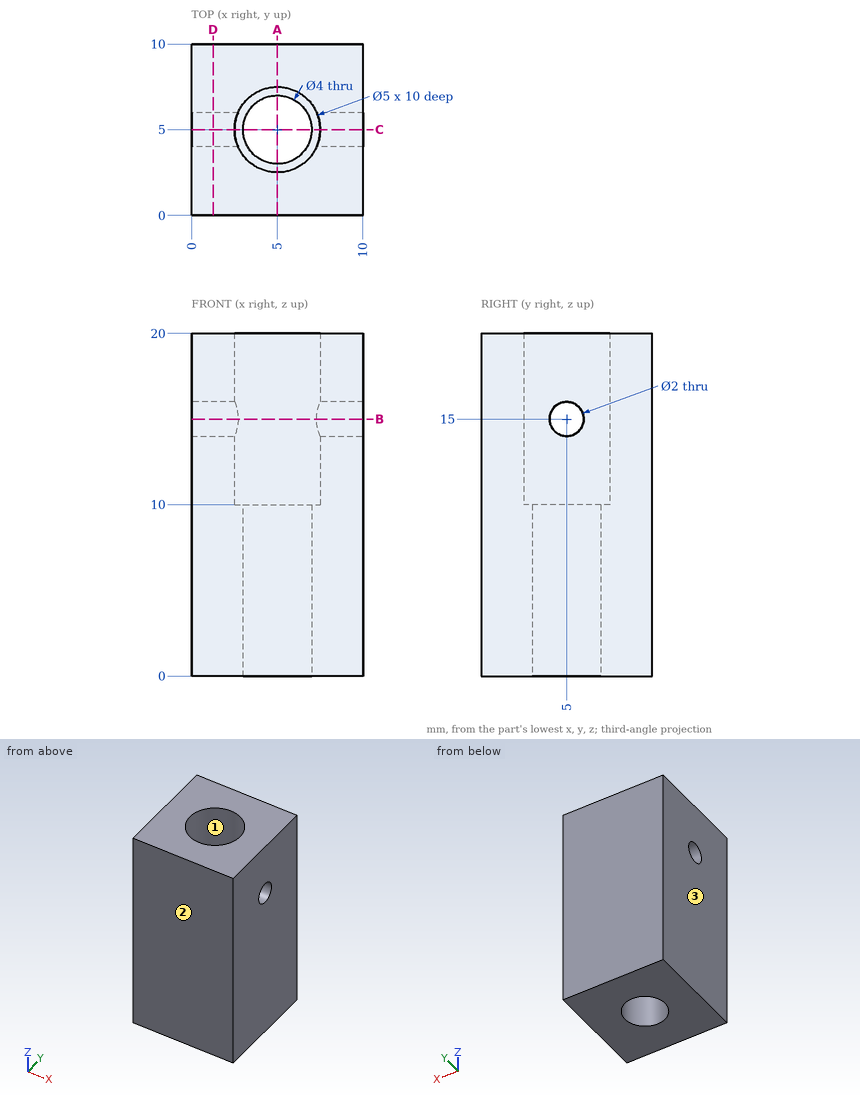
Design review of the part shown in the three views and the two pictorial views. Dimensions are in mm from the part's minimum x, y and z. Round coordinates to 2 decimals unless told otherwise and drop trailing zeros. Order: outer loops, then holes, each group sorted by start corner. A loop starts at its lowest first (then second) coordinate and runs counter-clockwise, first axis right, second up. Notation, with made-up numbers: (40.25, 64.5) - (57.25, 64.5) arc R24 ccw to (57.25, 81.5) - close; hole circle Ø8 at (-17.75, -36.5). An arc over 180 degrees is marked (long way). One line per question, with ' | ' between items.
Item 1: Take a section at B-B, the plane z = 15. Write out the cut boundary in (x, y).
Checks:
outline: (0, 0) - (10, 0) - (10, 4) - (7.29, 4) arc R2.5 cw to (2.71, 4) - (0, 4) - close; (0, 6) - (2.71, 6) arc R2.5 cw to (7.29, 6) - (10, 6) - (10, 10) - (0, 10) - close
Item 2: For P1, Ø6, axis at x = 3, z = 13.5, coming from the -Y side, flat-tipped, find the tip position at first contact; note if it passes through.
Checks:
P1: y = 0
Item 3: Wall thickness on line 1 (X direction, y = 6.5, z = 14.5); line 2 (Y direction, x = 8.35, z = 15); line 3 (Z direction, x = 1.8, y = 5): over which ranges is each line inside the solid? List them lowest first. Write a range as [from, to].
Checks:
line 1: [0, 3], [7, 10] | line 2: [0, 4], [6, 10] | line 3: [0, 14], [16, 20]
Item 4: Draft analysis for pull direction Y (two halves, no side actions). For the marked faces 1, 2 and 3, state which applies: +Y half, -Y half, draft (parallel to the pull), parting line (faces both ways), or undercut.
Checks:
face 1: undercut | face 2: -Y half | face 3: draft
Item 5: Take a section at C-C, the plane y = 5. Write out the cut boundary in (x, z).
Checks:
outline: (0, 0) - (3, 0) - (3, 10) - (2.5, 10) - (2.5, 14) - (0, 14) - close; (0, 16) - (2.5, 16) - (2.5, 20) - (0, 20) - close; (7, 0) - (10, 0) - (10, 14) - (7.5, 14) - (7.5, 10) - (7, 10) - close; (7.5, 16) - (10, 16) - (10, 20) - (7.5, 20) - close
Item 6: Take a section at A-A, the plane x = 5. Write out the cut boundary in (y, z), then the cut area to 3 significant figures.
Checks:
outline: (0, 0) - (3, 0) - (3, 10) - (2.5, 10) - (2.5, 20) - (0, 20) - close; (7, 0) - (10, 0) - (10, 20) - (7.5, 20) - (7.5, 10) - (7, 10) - close | area: 110 mm²
Item 7: Take a section at D-D, the plane x = 1.25. Write out the cut boundary in (y, z).
Checks:
outline: (0, 0) - (10, 0) - (10, 20) - (0, 20) - close; hole circle Ø2 at (5, 15)
